Part model, mm, in its own coordinate system. Face numbers are marked on the shaded views. A direction names the side the tool comes from. Coordinates: 2 decimals unless noted, no trailing zeros. Write each loop counter-clockwise with the first axis right and the second up, starting at its lowest first coordinate (ties: lowest second). Pieces come first, ordered by that corner, then holes. Notation, with made-up numbers: (16, 63.25) - (36, 63.25) arc R25 ccw to (36, 78.25) - close; hole circle Ø10 at (-12.5, 64). An arc over 180 degrees is marked (long way). Use a Markdown table: item, result.
```python
from build123d import *

# Parameters (mm, degrees)
SKETCH1_R                                           = 10
BOSS_EXTRUDE1_DEPTH                                 = 4
CBORE_FOR_M2_PAN_HEAD_SCREW1_D                      = 2.4
CBORE_FOR_M2_PAN_HEAD_SCREW1_CBORE_D                = 5
CBORE_FOR_M2_PAN_HEAD_SCREW1_CBORE_DEPTH            = 1.6
SKETCH4_R                                           = 2.25
BOSS_EXTRUDE2_DEPTH                                 = 6
CIRPATTERN1_COUNT                                   = 4
CSK_FOR_M3_COUNTERSUNK_FLAT_HEAD_SCREW1_D           = 3.4
CSK_FOR_M3_COUNTERSUNK_FLAT_HEAD_SCREW1_CSINK_D     = 6.3
CSK_FOR_M3_COUNTERSUNK_FLAT_HEAD_SCREW1_CSINK_ANGLE = 90
FILLET1_R                                           = 0.5


with BuildPart() as part:
    # Sketch1 → Boss-Extrude1 (new body)
    with BuildSketch(Plane(origin=(0, 0, 0), x_dir=(1, 0, 0), z_dir=(0, 1, 0))):
        with Locations(Location((0, 0, 0), (0, 0, 270))):
            Circle(SKETCH1_R)
    extrude(amount=BOSS_EXTRUDE1_DEPTH)

    # CBORE for M2 Pan Head Screw1 (through all)
    with Locations(Plane(origin=(0, 4, 0), x_dir=(1, 0, 0), z_dir=(0, 1, 0))):
        with Locations((6, 0)):
            cbore_for_m2_pan_head_screw1 = CounterBoreHole(CBORE_FOR_M2_PAN_HEAD_SCREW1_D / 2, CBORE_FOR_M2_PAN_HEAD_SCREW1_CBORE_D / 2, CBORE_FOR_M2_PAN_HEAD_SCREW1_CBORE_DEPTH)

    # Sketch4 → Boss-Extrude2 (add)
    with BuildSketch(Plane(origin=(0, 4, 0), x_dir=(1, 0, 0), z_dir=(0, 1, 0))):
        with Locations(Location((0, 0, 0), (0, 0, 270))):
            Circle(SKETCH4_R)
    extrude(amount=BOSS_EXTRUDE2_DEPTH)

    # CirPattern1: CBORE for M2 Pan Head Screw1 ×4 about axis
    cirpattern1_axis = Axis((0, 0, 0), (0, 1, 0))
    for i in range(1, CIRPATTERN1_COUNT):
        add(cbore_for_m2_pan_head_screw1.rotate(cirpattern1_axis, i * 360 / CIRPATTERN1_COUNT), mode=Mode.SUBTRACT)

    # CSK for M3 Countersunk Flat Head Screw1 (through all)
    with Locations(Plane.XZ):
        with Locations((0, 0)):
            CounterSinkHole(CSK_FOR_M3_COUNTERSUNK_FLAT_HEAD_SCREW1_D / 2, CSK_FOR_M3_COUNTERSUNK_FLAT_HEAD_SCREW1_CSINK_D / 2, counter_sink_angle=CSK_FOR_M3_COUNTERSUNK_FLAT_HEAD_SCREW1_CSINK_ANGLE)

    # Fillet1
    fillet1_edges = [part.edges().sort_by_distance(p)[0] for p in [
        (0, 4, -2.25),
    ]]
    fillet(fillet1_edges, radius=FILLET1_R)


solid = part.part
```
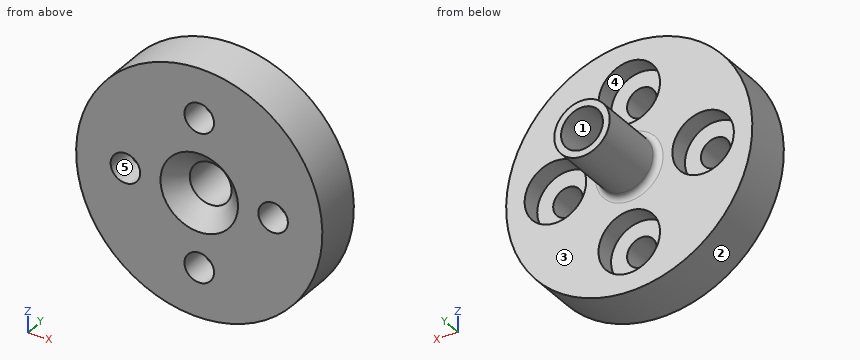
Item 1: Drop flat-ended pins along their axis: P1, Ø6.5, axis at x = 6, z = 0, coming from the +Y side; P2, Ø4, axis at x = 2.5, y = 3.5, coming from the +Z side; P3, Ø3, axis at y = 4, z = 2, coming from the +X side. Give the stop position or say it passes through.
From the geometry:
| item | result |
|---|---|
| P1 | y = 4 |
| P2 | z = 9.99 |
| P3 | x = 9.99 |
Item 2: Band-saw the part on C-C, the plane x = 0. Count the separate pieces of the cut face and the enclosed holes in it, then the cut area to 3 significant figures.
From the geometry:
| item | result |
|---|---|
| separate pieces | 4 |
| enclosed holes | 0 |
| area | 43.5 mm^2 |
Item 3: Two-plate mould, pull along X, no slides. Class the marked faces 1, 2 and 3: pulls with the +X half, pulls with the -X half, needs draft (parallel to the pull), parting line crosses it, or undercut.
From the geometry:
| item | result |
|---|---|
| face 1 | undercut |
| face 2 | parting line crosses it |
| face 3 | needs draft |
Item 4: Drill centre lines: probe 1 along X at (y, z) = (6.25, 0); probe 2 along Y at (x, z) = (2.75, 9.25); probe 3 along Z at (x, y) = (-0.25, 1). Where is each one in solid material? Low to high.
From the geometry:
| item | result |
|---|---|
| probe 1 | -2.25 to -1.7, 1.7 to 2.25 |
| probe 2 | 0 to 4 |
| probe 3 | -10 to -7.17, -4.83 to -2.14, 2.14 to 4.83, 7.17 to 10 |
Item 5: Which spindle directions (+Z, -Z, +X, -X, +Y, -Y) get a long thin tool onto all of the face, cutting with end or side? Do the marked faces 4 and 5. Say none if no direction does.
From the geometry:
| item | result |
|---|---|
| face 4 | +Y |
| face 5 | +Y, -Y |
Item 6: Band-saw the part on A-A, the plane z = -6. Give the cut face in (x, y), then the cut area to 3 significant figures.
From the geometry:
| item | result |
|---|---|
| outline | (-8, 0) - (-1.2, 0) - (-1.2, 2.4) - (-2.5, 2.4) - (-2.5, 4) - (-8, 4) - close; (1.2, 0) - (8, 0) - (8, 4) - (2.5, 4) - (2.5, 2.4) - (1.2, 2.4) - close |
| area | 50.2 mm^2 |
Item 7: Band-saw the part on B-B, the plane x = 6. Give the cut face in (y, z), then the cut area to 3 significant figures.
From the geometry:
| item | result |
|---|---|
| outline | (0, -8) - (4, -8) - (4, -2.5) - (2.4, -2.5) - (2.4, -1.2) - (0, -1.2) - close; (0, 1.2) - (2.4, 1.2) - (2.4, 2.5) - (4, 2.5) - (4, 8) - (0, 8) - close |
| area | 50.2 mm^2 |
Item 8: Band-saw the part on D-D, the plane y = 4.75. Give the cut face in (x, z).
From the geometry:
| item | result |
|---|---|
| outline | circle Ø4.5 at (0, 0); hole circle Ø3.4 at (0, 0) |
